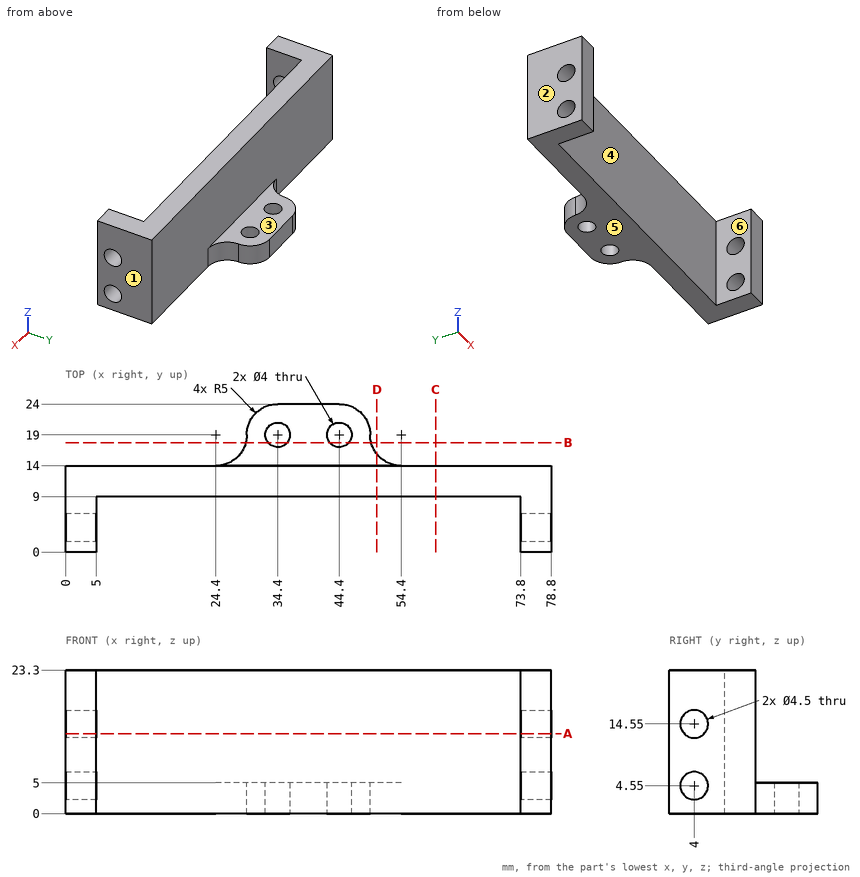
Verification items for this drawing (mm, ordinates from the low corner). A direction names the side the tool comes from. Give positions to 0.01 mm unless a question says otherwise; leave off trailing zeros. Write each loop counter-clockwise with the first axis right and the second up, starting at its lowest first coordinate (ties: lowest second). Pieces come first, ordered by that corner, then holes. Notation, with made-up numbers: (81, 66.5) - (95, 66.5) arc R16 ccw to (95, 73.5) - close; hole circle Ø10 at (65, 14.25). An arc over 180 degrees is marked (long way). Answer as a JSON object with one key per item and string values. Group by question number.
1) Sectioned sample at A-A (z = 13). Record the cut outline in (x, y), then the cut area to 3 significant figures.
2) Access from +Z, -Z, +X, -X, +Y, -Y to the whole of each face (thin tool, end or side, straight path). Record for the marked faces 5 and 6.
3) Sectioned sample at C-C (x = 60). Record the cut outline in (y, z), then the cut area to 4 significant figures.
4) Sectioned sample at B-B (y = 17.75). Record the cut outline in (x, z).
5) Sectioned sample at D-D (x = 50.5). Record the cut outline in (y, z).
6) Thickness scan on probe 1 along X at (y, z) = (2, 9.25); probe 2 along Y at (x, z) = (44.4, 2); probe 3 along Y at (x, z) = (8, 15.25). Record the ranges inside material, lowest first. Write a range as from..to.
7) Depth check by flat-ended pin: P1, Ø5, axis at x = 35.5, z = 19, coming from the -Y side; P2, Ø1.5, axis at x = 31.5, z = 10, coming from the +Y side; P3, Ø6.5, axis at x = 44.4, y = 19, coming from the +Z side. Enter the tip coordinate at first touch or a pass-through.
8) Release check for a two-part mould opening along X. For the marked faces 1, 2, 3 and 4 record: pulls with the +X half, pulls with the -X half, needs draft (parallel to the pull), parting line crosses it, or undercut.
Geometry results:
{
 "1": {"outline": "(0, 0) - (5, 0) - (5, 2.37) - (0, 2.37) - close; (0, 5.63) - (5, 5.63) - (5, 9) - (73.8, 9) - (73.8, 5.63) - (78.8, 5.63) - (78.8, 14) - (0, 14) - close; (73.8, 0) - (78.8, 0) - (78.8, 2.37) - (73.8, 2.37) - close", "area": "451 mm^2"},
 "2": {"face 5": "-Z, +X, -X, +Y, -Y", "face 6": "+Z, -Z, -Y"},
 "3": {"outline": "(9, 0) - (14, 0) - (14, 23.3) - (9, 23.3) - close", "area": "116.5 mm^2"},
 "4": {"outline": "(29.24, 0) - (32.84, 0) - (32.84, 5) - (29.24, 5) - close; (35.96, 0) - (42.84, 0) - (42.84, 5) - (35.96, 5) - close; (45.96, 0) - (49.56, 0) - (49.56, 5) - (45.96, 5) - close"},
 "5": {"outline": "(9, 0) - (15.87, 0) - (15.87, 5) - (14, 5) - (14, 23.3) - (9, 23.3) - close"},
 "6": {"probe 1": "x = 0..5, 73.8..78.8", "probe 2": "y = 9..17, 21..24", "probe 3": "y = 9..14"},
 "7": {"P1": "stops at y = 9", "P2": "stops at y = 14", "P3": "stops at z = 5"},
 "8": {"face 1": "pulls with the +X half", "face 2": "pulls with the -X half", "face 3": "needs draft", "face 4": "undercut"}
}
